For this review, take the finished solid that the model builds, in its own axes (mm). A direction names the side the tool comes from. Give positions to 0.01 mm unless a question says otherwise; leave off trailing zeros. Loops run counter-clockwise (first coordinate to the right, second up) from the corner with the lowest first, then second, coordinate; pieces in that order, holes last. Notation, with made-up numbers: (32, -1.75) - (80, -1.75) arc R35 ccw to (80, 35.25) - close; hole circle Ø8 at (19, -14). An arc over 180 degrees is marked (long way). Answer in a Markdown table with one row per item.
```python
from build123d import *

# Parameters (mm, degrees)
SKETCH1_W = 8
SKETCH1_H = 8


with BuildPart() as part:
    # Sketch1 → Revolve1 (revolve)
    with BuildSketch(Plane.XY, mode=Mode.PRIVATE) as revolve1_sk:
        with Locations((0, 6)):
            Rectangle(SKETCH1_W, SKETCH1_H)
    revolve(revolve1_sk.sketch.rotate(Axis((0, 0, 0), (1, 0, 0)), 90), axis=Axis((0, 0, 0), (1, 0, 0)))

    # Sketch2 → Cut-Revolve1 (revolve, cut)
    with BuildSketch(Plane.XY, mode=Mode.PRIVATE) as cut_revolve1_sk:
        Polygon((-4, 4.5), (-3.25, 4.5), (-3.25, 3.875), (4, 3.875), (4, 1.375), (-4, 1.375), align=None)
    revolve(cut_revolve1_sk.sketch.rotate(Axis((-4, 0, 0), (1, 0, 0)), 90), axis=Axis((-4, 0, 0), (1, 0, 0)), mode=Mode.SUBTRACT)

    # Sketch5 → Cut-Revolve2 (revolve, cut)
    with BuildSketch(Plane.XY, mode=Mode.PRIVATE) as cut_revolve2_sk:
        Polygon((-5.693293246, 11), (6.09167682, 11), (6.09167682, 9), (1.5, 9), (1.5, 7.5), (-1.5, 7.5), (-1.5, 9), (-5.693293246, 9), align=None)
    revolve(cut_revolve2_sk.sketch.rotate(Axis((-5.693293246, 0, 0), (1, 0, 0)), 90), axis=Axis((-5.693293246, 0, 0), (1, 0, 0)), mode=Mode.SUBTRACT)


solid = part.part
```
1. We need section A-A, the plane z = 0. Give the boundary of the cut face in (x, y) (3 decimals).
Values:
| item | result |
|---|---|
| outline | (-4, -9) - (-1.5, -9) - (-1.5, -7.5) - (1.5, -7.5) - (1.5, -9) - (4, -9) - (4, -3.875) - (-3.25, -3.875) - (-3.25, -4.5) - (-4, -4.5) - close; (-4, 4.5) - (-3.25, 4.5) - (-3.25, 3.875) - (4, 3.875) - (4, 9) - (1.5, 9) - (1.5, 7.5) - (-1.5, 7.5) - (-1.5, 9) - (-4, 9) - close |
2. We need section D-D, the plane z = -6.5. Give the boundary of the cut face in (x, y).
Values:
| item | result |
|---|---|
| outline | (-4, -6.22) - (-1.5, -6.22) - (-1.5, -3.74) - (1.5, -3.74) - (1.5, -6.22) - (4, -6.22) - (4, 6.22) - (1.5, 6.22) - (1.5, 3.74) - (-1.5, 3.74) - (-1.5, 6.22) - (-4, 6.22) - close |
3. Wall thickness on line 1 (X direction, y = -2.75, z = -7.25); line 2 (Y direction, x = -3.8, z = 0); line 3 (Y direction, x = -1.25, z = 0) (3 decimals): over which ranges is each line inside the solid? List them lowest first. Write a range as [from, to].
Values:
| item | result |
|---|---|
| line 1 | x = [-4, -1.5], [1.5, 4] |
| line 2 | y = [-9, -4.5], [4.5, 9] |
| line 3 | y = [-7.5, -3.875], [3.875, 7.5] |
4. Clearance check with flat-ended pins moving along their axes: pin 1 (4 mm diameter, centred on x = 1.5, y = -5.5, fed in from +Z); pin 2 (3 mm diameter, centred on y = 1, z = -2.5, fed in from -X); pin 3 (1.5 mm diameter, centred on x = -0.5, y = 0.5, fed in from +Z). State where each tip first meets the part, or that it passes through.
Values:
| item | result |
|---|---|
| pin 1 | stops at z = 8.29 |
| pin 2 | stops at x = -3.25 |
| pin 3 | stops at z = 7.5 |
5. For faces 4 (the face through (0.426, -3.842, -0.504)), 5 (the face through (1.5, -7.4, -2)), 6 (the face through (-3.25, -4, 1)), list the 3-axis set-ups (+Z, -Z, +X, -X, +Y, -Y) from which the entire face can be reached by the end or side of a thin tool; tool diameter is ignored.
Values:
| item | result |
|---|---|
| face 4 | +X, -X |
| face 5 | none |
| face 6 | -X |
6. Mouldability with a two-part tool opening along Z and no side actions: class faces 1 (the face through (-3.62, -3.04, -3.32)), 2 (the face through (-4, 4, -4)), 3 (the face through (-0.021, -6.324, 4.032)) as released by +Z, released by -Z, zero draft, split by the parting line, or undercut.
Values:
| item | result |
|---|---|
| face 1 | undercut |
| face 2 | zero draft |
| face 3 | split by the parting line |
7. We need section C-C, the plane x = -2. Give the boundary of the cut face in (y, z) (3 decimals), and give its area (3 significant figures).
Values:
| item | result |
|---|---|
| outline | circle Ø18 at (0, 0); hole circle Ø7.75 at (0, 0) |
| area | 207 mm^2 |
